Check sheet for the modelled part. Datum: model origin and axes. Units: mm. A direction names the side the tool comes from. Give positions to 0.01 mm unless a question says otherwise; leave off trailing zeros. Loops run counter-clockwise (first coordinate to the right, second up) from the corner with the lowest first, then second, coordinate; pieces in that order, holes last. Notation, with made-up numbers: M -39,6 L -2,6 A11 ccw -2,16 Z; hole C 46,68 d5. An arc over 180 degrees is marked long. Use one line per item in the form item = value.
from build123d import *

# Parameters (mm, degrees)
EXTRUDE_1_DEPTH     = 200
SKETCH_2_W          = 63
SKETCH_2_H          = 196
CUT_EXTRUDE_1_DEPTH = 17
SKETCH_4_W          = 67
SKETCH_4_H          = 17
EXTRUDE_2_DEPTH     = 5
CHAMFER_1_SIZE      = 5
FILLET_1_R          = 1
FILLET_3_R          = 1


with BuildPart() as part:
    # 草图1 → 凸台-拉伸1 (new body)
    with BuildSketch(Plane.XY):
        Polygon((-6, 28), (-73, 28), (-73, 32.656854249), (-78, 37.656854249), (-78, 38.928932188), (-73, 43.928932188), (-73, 47), (-6, 47), (-6, 43.928932188), (-1, 38.928932188), (-1, 37.656854249), (-6, 32.656854249), align=None)
    extrude(amount=-EXTRUDE_1_DEPTH)

    # 草图2 → 切除-拉伸1 (cut)
    with BuildSketch(Plane(origin=(0, 47, 0), x_dir=(1, 0, 0), z_dir=(0, 1, 0))):
        with Locations((-39.5, 100)):
            Rectangle(SKETCH_2_W, SKETCH_2_H)
    extrude(amount=-CUT_EXTRUDE_1_DEPTH, mode=Mode.SUBTRACT)

    # 草图4 → 凸台-拉伸2 (add)
    with BuildSketch(Plane.XY):
        with Locations((-39.5, 47.5)):
            Rectangle(SKETCH_4_W, SKETCH_4_H)
    extrude(amount=EXTRUDE_2_DEPTH)

    # 倒角1
    chamfer_1_edges = [part.edges().sort_by_distance(p)[0] for p in [
        (-73, 39, 2.5),
        (-6, 39, 2.5),
    ]]
    chamfer(chamfer_1_edges, length=CHAMFER_1_SIZE)

    # 圆角1
    fillet_1_edges = [part.edges().sort_by_distance(p)[0] for p in [
        (-68, 39, 2.5),
        (-73, 44, -97.5),
        (-11, 39, 2.5),
        (-6, 44, -97.5),
        (-6, 56, 2.5),
        (-73, 56, 2.5),
    ]]
    fillet(fillet_1_edges, radius=FILLET_1_R)

    # 圆角3
    fillet_3_edges = [part.edges().sort_by_distance(p)[0] for p in [
        (-75.5, 35.156854249, 0),
        (-75.457984297, 41.470947892, 0),
        (-78, 38.292893219, 0),
        (-75.5, 35.156854249, -200),
        (-78, 38.292893219, -200),
        (-75.457984297, 41.470947892, -200),
        (-3.5, 35.156854249, -200),
        (-1, 38.292893219, -200),
        (-3.542015703, 41.470947892, -200),
        (-3.5, 35.156854249, 0),
        (-1, 38.292893219, 0),
        (-3.542015703, 41.470947892, 0),
    ]]
    fillet(fillet_3_edges, radius=FILLET_3_R)


solid = part.part
1) Section check B-B (z = -119.5). Record the cut outline in (x, y), then the cut area to 3 significant figures.
Evaluation:
outline = M -78,37.66 L -73,32.66 L -73,28 L -6,28 L -6,32.66 L -1,37.66 L -1,38.93 L -6.08,44.01 A1 ccw -6,44.41 L -6,47 L -8,47 L -8,30 L -71,30 L -71,47 L -73,47 L -73,44.41 A1 ccw -72.92,44.01 L -78,38.93 Z
area = 265 mm^2
2) Section check C-C (y = 52.75). Record the cut outline in (x, z).
Evaluation:
outline = M -73,0 L -6,0 L -6,5 L -73,5 Z
3) Release check for a two-part mould opening along X. For faces 6 (the face through (-73, 46.5, -90.4)), 7 (the face through (-71, 39, -99)), 8 (the face through (-6, 46.5, -90.4)) record: pulls with the +X half, pulls with the -X half, needs draft (parallel to the pull), parting line crosses it, or undercut.
Evaluation:
face_6 = pulls with the -X half
face_7 = undercut
face_8 = pulls with the +X half
4) Set-up check for faces 1 (the face through (-3.465, 35.192, -98.614)), 2 (the face through (-40, 52, 0)), 3 (the face through (-40, 39, 2)), 4 (the face through (-75.322, 35.404, -199.715)), 5 (the face through (-40, 30, -101)): record each of +Z, -Z, +X, -X, +Y, -Y from which the full face is reachable in a straight line by a thin tool's end or side.
Evaluation:
face_1 = +Z, -Z, +X, -Y
face_2 = -Z, +X, -X, +Y
face_3 = +Z, +X, -X, -Y
face_4 = -Z, -X, -Y
face_5 = +Y
5) Depth check by flat-ended pin: pin 1 Ø5.5 at (y, z) = (48.5, -60.5) entering from +X; pin 2 Ø4 at (x, z) = (-23.5, -31) entering from +Y; pin 3 Ø6.5 at (y, z) = (30.5, -126) entering from +X. Enter the tip coordinate at first touch or a pass-through.
Evaluation:
pin_1 = -6
pin_2 = 30
pin_3 = -4.91
6) Section check A-A (x = -17). Record the cut outline in (y, z), then the cut area to 3 significant figures.
Evaluation:
outline = M 28,-200 L 47,-200 L 47,-198 L 30,-198 L 30,-2 L 47,-2 L 47,0 L 56,0 L 56,5 L 39,5 L 39,0 L 28,0 Z
area = 553 mm^2
7) Scan lines: line 1 (Z direction, x = -27, y = 31.75); line 2 (Z direction, x = -33, y = 45.5); line 3 (X direction, y = 45.25, z = -181.5). Record each from-to range of solid material in increasing order.
Evaluation:
line_1 = -200 to -198, -2 to 0
line_2 = -200 to -198, -2 to 5
line_3 = -73 to -71, -8 to -6
